Read the model definition and answer for the solid it produces. Units are mm, in the model's axes. Coordinates: 2 decimals unless noted, no trailing zeros. Loops run counter-clockwise (first coordinate to the right, second up) from the corner with the lowest first, then second, coordinate; pieces in that order, holes last. Notation, with made-up numbers: (23, 60) -> (49, 60) arc R13 ccw to (49, 75) -> close; hole circle Ø10 at (-3, -8). An arc over 180 degrees is marked (long way). Answer in a Markdown table with one row per item.
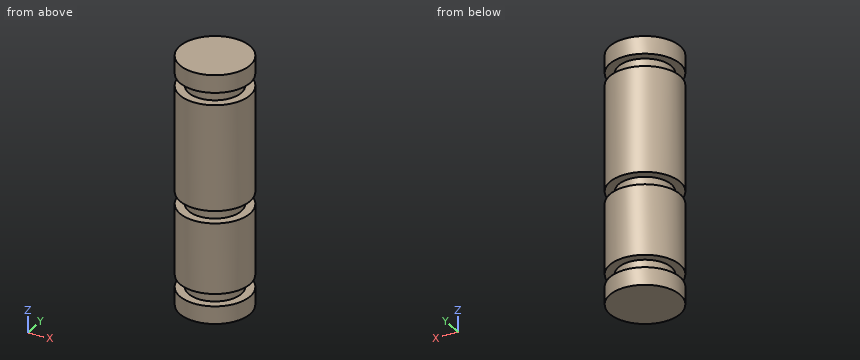
```python
from build123d import *

# Parameters (mm, degrees)
ESBO_O1_R                = 2
RESSALTO_EXTRUS_O1_DEPTH = 1
ESBO_O2_R                = 1.5
RESSALTO_EXTRUS_O2_DEPTH = 0.7
ESBO_O3_R                = 2
RESSALTO_EXTRUS_O3_DEPTH = 4
ESBO_O4_R                = 1.5
RESSALTO_EXTRUS_O4_DEPTH = 0.7
ESBO_O5_R                = 2
RESSALTO_EXTRUS_O5_DEPTH = 6
ESBO_O6_R                = 1.5
RESSALTO_EXTRUS_O6_DEPTH = 0.7
ESBO_O7_R                = 2
RESSALTO_EXTRUS_O7_DEPTH = 1


with BuildPart() as part:
    # Esboço1 → Ressalto-extrusão1 (new body)
    with BuildSketch(Plane.XY):
        Circle(ESBO_O1_R)
    extrude(amount=RESSALTO_EXTRUS_O1_DEPTH)

    # Esboço2 → Ressalto-extrusão2 (add)
    with BuildSketch(Plane.XY.offset(1)):
        Circle(ESBO_O2_R)
    extrude(amount=RESSALTO_EXTRUS_O2_DEPTH)

    # Esboço3 → Ressalto-extrusão3 (add)
    with BuildSketch(Plane.XY.offset(1.7)):
        Circle(ESBO_O3_R)
    extrude(amount=RESSALTO_EXTRUS_O3_DEPTH)

    # Esboço4 → Ressalto-extrusão4 (add)
    with BuildSketch(Plane.XY.offset(5.7)):
        Circle(ESBO_O4_R)
    extrude(amount=RESSALTO_EXTRUS_O4_DEPTH)

    # Esboço5 → Ressalto-extrusão5 (add)
    with BuildSketch(Plane.XY.offset(6.4)):
        Circle(ESBO_O5_R)
    extrude(amount=RESSALTO_EXTRUS_O5_DEPTH)

    # Esboço6 → Ressalto-extrusão6 (add)
    with BuildSketch(Plane.XY.offset(12.4)):
        Circle(ESBO_O6_R)
    extrude(amount=RESSALTO_EXTRUS_O6_DEPTH)

    # Esboço7 → Ressalto-extrusão7 (add)
    with BuildSketch(Plane.XY.offset(13.1)):
        Circle(ESBO_O7_R)
    extrude(amount=RESSALTO_EXTRUS_O7_DEPTH)


solid = part.part
```
1. A cutting plane is placed at C-C on x = -1.7. Give the vertices of the cut face in (y, z).
A:
| item | result |
|---|---|
| outline | (-1.05, 0) -> (1.05, 0) -> (1.05, 1) -> (-1.05, 1) -> close; (-1.05, 1.7) -> (1.05, 1.7) -> (1.05, 5.7) -> (-1.05, 5.7) -> close; (-1.05, 6.4) -> (1.05, 6.4) -> (1.05, 12.4) -> (-1.05, 12.4) -> close; (-1.05, 13.1) -> (1.05, 13.1) -> (1.05, 14.1) -> (-1.05, 14.1) -> close |
2. Find the intervals of material crossed by probe 1 along Z at (x, y) = (-1.8, -0.6); probe 2 along Y at (x, z) = (0.1, 9); probe 3 along X at (y, z) = (0.15, 1.75), in increasing order.
A:
| item | result |
|---|---|
| probe 1 | z = 0 to 1, 1.7 to 5.7, 6.4 to 12.4, 13.1 to 14.1 |
| probe 2 | y = -2 to 2 |
| probe 3 | x = -1.99 to 1.99 |
3. A cutting plane is placed at A-A on x = 0. Give the vertices of the cut face in (y, z).
A:
| item | result |
|---|---|
| outline | (-2, 0) -> (2, 0) -> (2, 1) -> (1.5, 1) -> (1.5, 1.7) -> (2, 1.7) -> (2, 5.7) -> (1.5, 5.7) -> (1.5, 6.4) -> (2, 6.4) -> (2, 12.4) -> (1.5, 12.4) -> (1.5, 13.1) -> (2, 13.1) -> (2, 14.1) -> (-2, 14.1) -> (-2, 13.1) -> (-1.5, 13.1) -> (-1.5, 12.4) -> (-2, 12.4) -> (-2, 6.4) -> (-1.5, 6.4) -> (-1.5, 5.7) -> (-2, 5.7) -> (-2, 1.7) -> (-1.5, 1.7) -> (-1.5, 1) -> (-2, 1) -> close |
4. A cutting plane is placed at D-D on z = 11.75. Give the vertices of the cut face in (x, y).
A:
| item | result |
|---|---|
| outline | circle Ø4 at (0, 0) |
